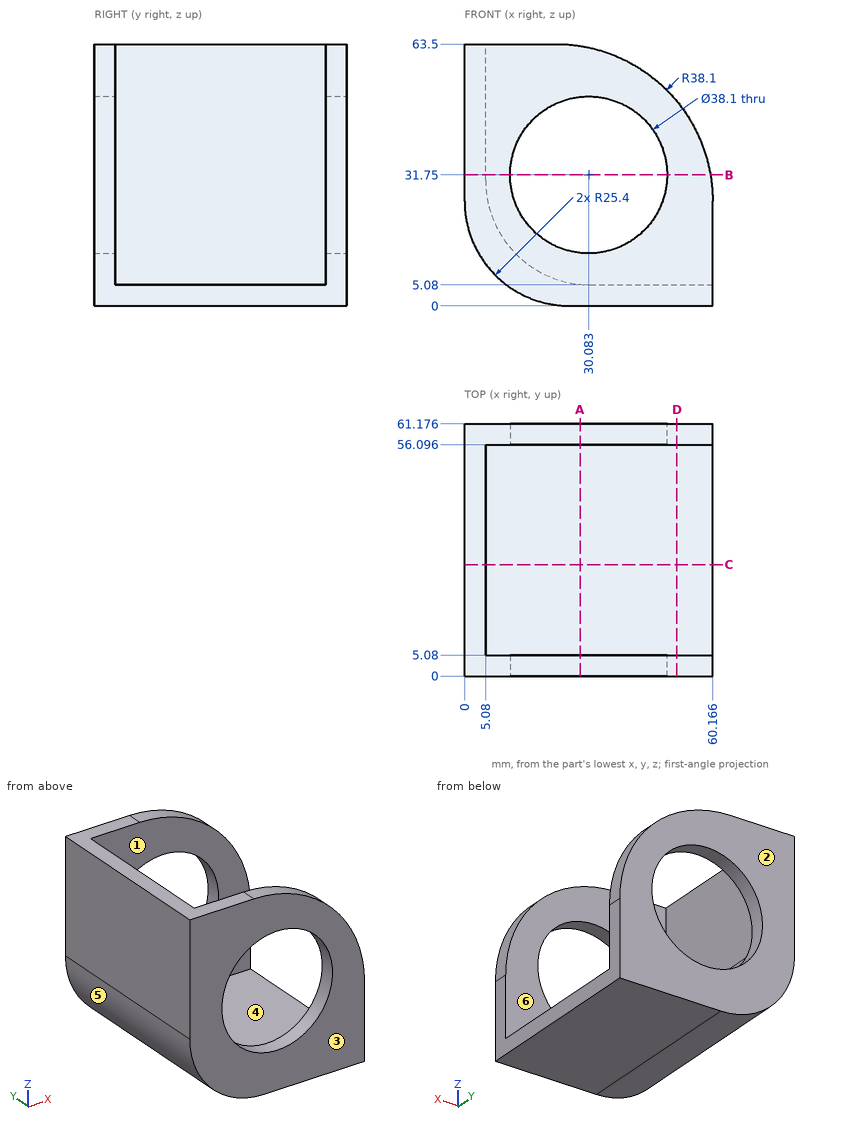
Source: three-view drawing plus pictorial views. Frame: mm from the lowest corner of the part. A direction names the side the tool comes from. Coordinates: 2 decimals unless noted, no trailing zeros. Write each loop counter-clockwise with the first axis right and the second up, starting at its lowest first coordinate (ties: lowest second). Pieces come first, ordered by that corner, then holes. Notation, with made-up numbers: (1.5, -24) -> (35.5, -24) arc R12 cw to (35.5, -19) -> close; hole circle Ø7 at (18.25, 34). An arc over 180 degrees is marked (long way). Write each question's results on one line, items separated by ' | '.
Item 1: Section query A-A on x = 28. Return loops of the section in (y, z) (1 decimal), plus the area to 3 significant figures.
Conclusion:
outline: (0, 0) -> (61.2, 0) -> (61.2, 12.8) -> (56.1, 12.8) -> (56.1, 5.2) -> (5.1, 5.2) -> (5.1, 12.8) -> (0, 12.8) -> close; (0, 50.7) -> (5.1, 50.7) -> (5.1, 63) -> (0, 63) -> close; (56.1, 50.7) -> (61.2, 50.7) -> (61.2, 63) -> (56.1, 63) -> close | area: 521 mm^2
Item 2: Pin query (flat end, axial travel): pin 1 Ø10 at (x, z) = (30.5, 42.5) entering from +Y; pin 2 Ø23.5 at (x, y) = (38.5, 26.5) entering from +Z (1 decimal); pin 3 Ø16.5 at (y, z) = (31.5, 42.5) entering from +X; pin 4 Ø2 at (x, y) = (12.5, 22.5) entering from +Z. Return the tip coordinate at first contact, or that it passes through.
Conclusion:
pin 1: passes through | pin 2: stops at z = 5.4 | pin 3: stops at x = 5.08 | pin 4: stops at z = 13.6
Item 3: Section query B-B on z = 31.75. Return loops of the section in (x, y).
Conclusion:
outline: (0, 0) -> (11.03, 0) -> (11.03, 5.08) -> (5.08, 5.08) -> (5.08, 56.1) -> (11.03, 56.1) -> (11.03, 61.18) -> (0, 61.18) -> close; (49.13, 0) -> (59.63, 0) -> (59.63, 5.08) -> (49.13, 5.08) -> close; (49.13, 56.1) -> (59.63, 56.1) -> (59.63, 61.18) -> (49.13, 61.18) -> close
Item 4: Set-up query: the marked faces 5 and 6. Return all of +Z, -Z, +X, -X, +Y, -Y with unobstructed straight access to the full face (end or side cutting, diameter ignored); none if empty.
Conclusion:
face 5: -Z, -X, +Y, -Y | face 6: +Z, +X
Item 5: Section query D-D on x = 51.5. Return loops of the section in (y, z), plus the area to 3 significant figures.
Conclusion:
outline: (0, 0) -> (61.18, 0) -> (61.18, 49.59) -> (56.1, 49.59) -> (56.1, 5.08) -> (5.08, 5.08) -> (5.08, 49.59) -> (0, 49.59) -> close | area: 763 mm^2
Item 6: Material intervals for probe 1 along Y at (x, z) = (48, 7.5); probe 2 along Z at (x, y) = (56, 31), sorted ascending.
Conclusion:
probe 1: y = 0 to 5.08, 56.1 to 61.18 | probe 2: z = 0 to 5.08
Item 7: Section query C-C on y = 27. Return loops of the section in (x, z).
Conclusion:
outline: (0, 25.4) arc R25.4 ccw to (25.4, 0) -> (60.17, 0) -> (60.17, 5.08) -> (30.48, 5.08) arc R25.4 cw to (5.08, 30.48) -> (5.08, 63.5) -> (0, 63.5) -> close
Item 8: Mould query, pull axis Y, two halves, no side actions, for the marked faces 1, 2, 3 and 4. Classes: +Y half, -Y half, draft (parallel to the pull), parting line (faces both ways), or undercut.
Conclusion:
face 1: undercut | face 2: +Y half | face 3: -Y half | face 4: undercut
